from build123d import *

# Parameters (mm, degrees)
F1_DEPTH = 25.4
F3_DEPTH = 96.466142
F4_W     = 12.7
F4_H     = 44.147057
F5_DEPTH = 101.372375
F6_R     = 6.35
F7_DEPTH = 25.401
F9_DEPTH = 31.75


with BuildPart() as f1:
    # F0 (on Front) → F1 (new body)
    with BuildSketch(Plane.XZ):
        Polygon((0, 82.55), (0, 0), (101.371375, 0), (101.371375, 44.147057), (50.8, 82.55), align=None)
    extrude(amount=F1_DEPTH)

    # F2 (on face) → F3 (cut, through all)
    with BuildSketch(Plane(origin=(58.339296, 0, 76.824801), x_dir=(0.7964, 0, -0.604771), z_dir=(0.604771, 0, 0.7964))):
        Polygon((36.194164, 0), (54.033275, -12.7), (54.033275, 0), align=None)
    extrude(amount=-F3_DEPTH, mode=Mode.SUBTRACT)

    # F4 (on face) → F5 (cut, through all)
    with BuildSketch(Plane.YZ.offset(101.371375)):
        with Locations((-6.35, 22.073528)):
            Rectangle(F4_W, F4_H)
    extrude(amount=-F5_DEPTH, mode=Mode.SUBTRACT)

    # F6 (on face) → F7 (cut, through all)
    with BuildSketch(Plane.XZ.offset(25.4)):
        with Locations((25.4, 69.85)):
            Circle(F6_R)
    extrude(amount=-F7_DEPTH, mode=Mode.SUBTRACT)

    # F8 (on face) → F9 (join)
    with BuildSketch(Plane.XZ.offset(25.4)):
        Polygon((50.685688, 31.75), (0, 31.75), (0, 6.35), (6.35, 6.35), (6.35, 0), (50.685688, 0), (50.685688, 12.7), (63.385688, 12.7), (63.385688, 19.05), (50.685688, 19.05), align=None)
    extrude(amount=F9_DEPTH)


solid = f1.part
Geometry: final body of the model. Coordinates: model frame, mm. A direction names the side the tool comes from. Give positions to 0.01 mm unless a question says otherwise; leave off trailing zeros. Order: outer loops, then holes, each group sorted by start corner. A loop starts at its lowest first (then second) coordinate and runs counter-clockwise, first axis right, second up. Notation, with made-up numbers: (62, 81) -> (102, 81) arc R29 ccw to (102, 114) -> close; hole circle Ø10 at (64.25, 7). An arc over 180 degrees is marked (long way). Answer as a JSON object with one key per item and string values.
Q1. Section C-C (z = 69.85). Output: boundary loops of the cut face in (x, y).
Entries:
{"outline": "(0, -25.4) -> (19.05, -25.4) -> (19.05, 0) -> (0, 0) -> close; (31.75, -25.4) -> (67.52, -25.4) -> (67.52, 0) -> (31.75, 0) -> close"}
Q2. Access query for faces 1 (the flat face through (3, -25.4, 3)), 2 (the flat face through (51, -6, 44.147)), 3 (the flat face through (26, -41, 31.75)), 4 (the flat face through (50.686, -41, 25)). Directions: +Z, -Z, +X, -X, +Y, -Y. A direction counts if a zero-diameter tool reaches every point of the face in a straight line with its end or side. Return the directions, or none.
Entries:
{"face 1": "-Z, -X, -Y", "face 2": "-Z, +X, -X, +Y", "face 3": "+Z, +X, -X, -Y", "face 4": "+Z, +X, -Y"}
Q3. Section B-B (y = -28). Output: boundary loops of the cut face in (x, z), plus the area to 3 significant figures.
Entries:
{"outline": "(0, 6.35) -> (6.35, 6.35) -> (6.35, 0) -> (50.69, 0) -> (50.69, 12.7) -> (63.39, 12.7) -> (63.39, 19.05) -> (50.69, 19.05) -> (50.69, 31.75) -> (0, 31.75) -> close", "area": "1,650 mm^2"}
Q4. Material intervals for probe 1 along Z at (x, y) = (25.4, -14.25); probe 2 along Z at (x, y) = (16, -48.5); probe 3 along Y at (x, z) = (58.5, 23), sorted ascending.
Entries:
{"probe 1": "z = 0 to 63.5, 76.2 to 82.55", "probe 2": "z = 0 to 31.75", "probe 3": "y = -25.4 to -12.7"}
Q5. Section A-A (x = 25.4). Output: boundary loops of the cut face in (y, z), plus the area to 3 significant figures.
Entries:
{"outline": "(-57.15, 0) -> (-12.7, 0) -> (-12.7, 44.15) -> (0, 44.15) -> (0, 63.5) -> (-25.4, 63.5) -> (-25.4, 31.75) -> (-57.15, 31.75) -> close; (-25.4, 76.2) -> (0, 76.2) -> (0, 82.55) -> (-25.4, 82.55) -> close", "area": "2,220 mm^2"}
Q6. Section D-D (z = 17). Output: boundary loops of the cut face in (x, y).
Entries:
{"outline": "(0, -57.15) -> (63.39, -57.15) -> (63.39, -25.4) -> (101.37, -25.4) -> (101.37, -12.7) -> (0, -12.7) -> close"}
Q7. First-contact query: pin 1 (4 mm diameter, centred on x = 56, y = -43, fed in from -Z); pin 2 (8 mm diameter, centred on x = 80.5, z = 26.5, fed in from +Y); pin 3 (6.5 mm diameter, centred on y = -36, z = 7.5, fed in from +X); pin 4 (2 mm diameter, centred on y = -26.5, z = 47, fed in from +X). Flat tips, straight axial feed; report the tip coordinate or a pass-through.
Entries:
{"pin 1": "stops at z = 12.7", "pin 2": "stops at y = -12.7", "pin 3": "stops at x = 50.69", "pin 4": "passes through"}
Q8. Draft query along X for faces 5 (the cylindrical face through (24.573, -12.878, 76.146)), 6 (the flat face through (63.386, -41, 16)), 7 (the flat face through (0, -22, 42)). Return one class per face: released by +X, released by -X, zero draft, split by the parting line, or undercut.
Entries:
{"face 5": "undercut", "face 6": "released by +X", "face 7": "released by -X"}
